Geometry check sheet. Reference: the model listing, model coordinates, mm. Give positions to 0.01 mm unless a question says otherwise; leave off trailing zeros. Write each loop counter-clockwise with the first axis right and the second up, starting at its lowest first coordinate (ties: lowest second). Pieces come first, ordered by that corner, then holes. Notation, with made-up numbers: (-11, 83) -> (22, 83) arc R22 ccw to (22, 92) -> close; hole circle Ø3 at (50.5, -10.75). An arc over 180 degrees is marked (long way). Use a Markdown table: item, result. Add a question column.
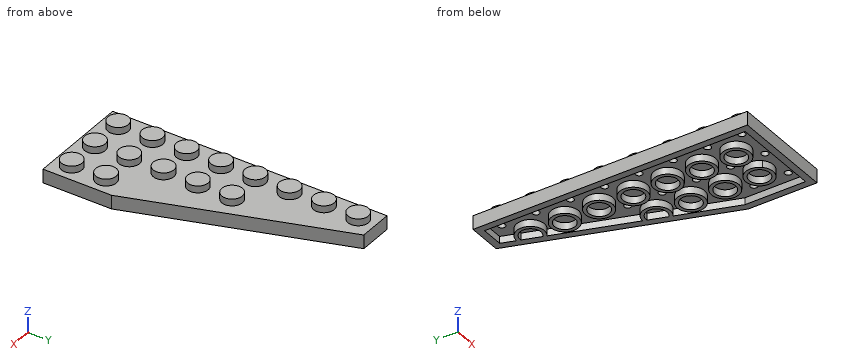
from build123d import *

# Parameters (mm, degrees)
F0_R     = 2.38125
F1_DEPTH = 3.175
F2_DEPTH = 4.7625
F3_T     = -1.5875
F4_R     = 3.175
F4_R_2   = 2.38125
F5_DEPTH = 1.5875


with BuildPart() as f1:
    # F0 (on Top) → F1 (new body)
    with BuildSketch(Plane.XY):
        Polygon((-3.96875, 31.75), (-11.90625, 31.75), (-11.90625, -31.75), (11.90625, -31.75), (11.90625, -15.875), align=None)
        with Locations((-7.9375, -27.78125)):
            Circle(F0_R, mode=Mode.SUBTRACT)
        with Locations((-7.9375, -19.84375)):
            Circle(F0_R, mode=Mode.SUBTRACT)
        with Locations((-7.9375, -11.90625)):
            Circle(F0_R, mode=Mode.SUBTRACT)
        with Locations((-7.9375, -3.96875)):
            Circle(F0_R, mode=Mode.SUBTRACT)
        with Locations((0, -27.78125)):
            Circle(F0_R, mode=Mode.SUBTRACT)
        with Locations((0, -19.84375)):
            Circle(F0_R, mode=Mode.SUBTRACT)
        with Locations((7.9375, -27.78125)):
            Circle(F0_R, mode=Mode.SUBTRACT)
        with Locations((7.9375, -19.84375)):
            Circle(F0_R, mode=Mode.SUBTRACT)
        with Locations((0, -11.90625)):
            Circle(F0_R, mode=Mode.SUBTRACT)
        with Locations((0, -3.96875)):
            Circle(F0_R, mode=Mode.SUBTRACT)
        with Locations((-7.9375, 3.96875)):
            Circle(F0_R, mode=Mode.SUBTRACT)
        with Locations((-7.9375, 11.90625)):
            Circle(F0_R, mode=Mode.SUBTRACT)
        with Locations((-7.9375, 19.84375)):
            Circle(F0_R, mode=Mode.SUBTRACT)
        with Locations((-7.9375, 27.78125)):
            Circle(F0_R, mode=Mode.SUBTRACT)
        with Locations((0, 3.96875)):
            Circle(F0_R, mode=Mode.SUBTRACT)
    extrude(amount=F1_DEPTH)

    # F0 (on Top) → F2 (join)
    with BuildSketch(Plane.XY):
        with Locations((-7.9375, 27.78125)):
            Circle(F0_R)
        with Locations((-7.9375, 19.84375)):
            Circle(F0_R)
        with Locations((-7.9375, 11.90625)):
            Circle(F0_R)
        with Locations((-7.9375, 3.96875)):
            Circle(F0_R)
        with Locations((-7.9375, -3.96875)):
            Circle(F0_R)
        with Locations((-7.9375, -11.90625)):
            Circle(F0_R)
        with Locations((-7.9375, -19.84375)):
            Circle(F0_R)
        with Locations((-7.9375, -27.78125)):
            Circle(F0_R)
        with Locations((0, -27.78125)):
            Circle(F0_R)
        with Locations((0, -19.84375)):
            Circle(F0_R)
        with Locations((0, -11.90625)):
            Circle(F0_R)
        with Locations((0, -3.96875)):
            Circle(F0_R)
        with Locations((0, 3.96875)):
            Circle(F0_R)
        with Locations((7.9375, -19.84375)):
            Circle(F0_R)
        with Locations((7.9375, -27.78125)):
            Circle(F0_R)
    extrude(amount=F2_DEPTH)

    # F3
    f3_openings = [f1.faces().sort_by_distance(p)[0] for p in [
        (-2.204861, -5.291667, 0),
    ]]
    offset(amount=F3_T, openings=f3_openings, kind=Kind.INTERSECTION)

    # F4 (on face) → F5 (join)
    with BuildSketch(Plane(origin=(0, 0, 1.5875), x_dir=(1, 0, 0), z_dir=(0, 0, -1))):
        with BuildLine():
            ThreePointArc((1.7236859697, 26.0575640303), (1.7236859697, 21.5674359697), (6.2138140303, 21.5674359697))
            Line((6.2138140303, 21.5674359697), (5.6525480227, 22.1287019773))
            ThreePointArc((5.6525480227, 22.1287019773), (2.2849519773, 22.1287019773), (2.2849519773, 25.4962980227))
            Line((2.2849519773, 25.4962980227), (1.7236859697, 26.0575640303))
        make_face()
        with BuildLine():
            Line((5.6525480227, 22.1287019773), (6.2138140303, 21.5674359697))
            ThreePointArc((6.2138140303, 21.5674359697), (6.9020675157, 22.5974801022), (7.14375, 23.8125))
            ThreePointArc((7.14375, 23.8125), (5.1837698978, 26.7458175157), (1.7236859697, 26.0575640303))
            Line((1.7236859697, 26.0575640303), (2.2849519773, 25.4962980227))
            ThreePointArc((2.2849519773, 25.4962980227), (4.8800149233, 26.0124881368), (6.35, 23.8125))
            ThreePointArc((6.35, 23.8125), (6.1687381368, 22.9012350767), (5.6525480227, 22.1287019773))
        make_face()
        with Locations((3.96875, 15.875)):
            Circle(F4_R)
        with Locations((3.96875, 15.875)):
            Circle(F4_R_2, mode=Mode.SUBTRACT)
        with Locations((3.96875, 7.9375)):
            Circle(F4_R)
        with Locations((3.96875, 7.9375)):
            Circle(F4_R_2, mode=Mode.SUBTRACT)
        with BuildLine():
            Line((5.5381726179, 1.7908836392), (5.8046687532, 2.590372045))
            ThreePointArc((5.8046687532, 2.590372045), (0.9566805287, 1.0040231571), (3.8832617755, -3.1738488879))
            Line((3.8832617755, -3.1738488879), (4.1497579108, -2.3743604821))
            ThreePointArc((4.1497579108, -2.3743604821), (1.7096978965, 0.7530173678), (5.5381726179, 1.7908836392))
        make_face()
        with BuildLine():
            Line((-2.3993273821, -22.0216163608), (-2.1328312468, -21.222127955))
            ThreePointArc((-2.1328312468, -21.222127955), (-6.9808194713, -22.8084768429), (-4.0542382245, -26.9863488879))
            Line((-4.0542382245, -26.9863488879), (-3.7877420892, -26.1868604821))
            ThreePointArc((-3.7877420892, -26.1868604821), (-6.2278021035, -23.0594826322), (-2.3993273821, -22.0216163608))
        make_face()
        with Locations((-3.96875, 23.8125)):
            Circle(F4_R)
        with Locations((-3.96875, 23.8125)):
            Circle(F4_R_2, mode=Mode.SUBTRACT)
        with Locations((-3.96875, 15.875)):
            Circle(F4_R)
        with Locations((-3.96875, 15.875)):
            Circle(F4_R_2, mode=Mode.SUBTRACT)
        with Locations((-3.96875, 7.9375)):
            Circle(F4_R)
        with Locations((-3.96875, 7.9375)):
            Circle(F4_R_2, mode=Mode.SUBTRACT)
        with Locations((-3.96875, 0)):
            Circle(F4_R)
        with Locations((-3.96875, 0)):
            Circle(F4_R_2, mode=Mode.SUBTRACT)
        with Locations((-3.96875, -7.9375)):
            Circle(F4_R)
        with Locations((-3.96875, -7.9375)):
            Circle(F4_R_2, mode=Mode.SUBTRACT)
        with Locations((-3.96875, -15.875)):
            Circle(F4_R)
        with Locations((-3.96875, -15.875)):
            Circle(F4_R_2, mode=Mode.SUBTRACT)
    extrude(amount=F5_DEPTH)


solid = f1.part
1) Material ranges on probe 1 along Y at (x, z) = (-1.5, 4.35); probe 2 along X at (y, z) = (0, 0.55); probe 3 along X at (y, z) = (-15, 1.3), recorded low to high. Write a range as [from, to].
2) Gauge pin test, flat ends, axial feed: P1, Ø1.4, axis at x = -4, y = 8.5, coming from the -Z side; P2, Ø1, axis at x = 0, y = -3.97, coming from the -Z side (3 decimals); P3, Ø1.7, axis at y = 0.5, z = 1, coming from the +X side. Record the tip position at first contact, or that the pin passes through.
3) Sectioned sample at B-B, the plane y = 24. Enter the section's corners in (x, z) (1 decimal).
Check values:
| question | item | result |
|---|---|---|
| 1 | probe 1 | [-29.63, -25.93], [-21.69, -17.99], [-13.76, -10.06], [-5.82, -2.12], [2.12, 5.82] |
| 1 | probe 2 | [-11.91, -10.32], [-7.14, -6.35], [-1.59, -0.79], [0.79, 1.59], [4.94, 6.61] |
| 1 | probe 3 | [-11.91, -10.32], [-7.02, -6.18], [-1.75, -0.92], [0.92, 1.75], [6.18, 7.02], [9.94, 11.61] |
| 2 | P1 | z = 1.59 |
| 2 | P2 | z = 3.175 |
| 2 | P3 | x = 6.73 |
| 3 | outline | (-11.9, 0) -> (-10.3, 0) -> (-10.3, 1.6) -> (-7.1, 1.6) -> (-7.1, 0) -> (-6.3, 0) -> (-6.3, 1.6) -> (-3.1, 1.6) -> (-3.1, 0) -> (-1.4, 0) -> (-1.4, 3.2) -> (-11.9, 3.2) -> close |
